Read the model definition and answer for the solid it produces. Units are mm, in the model's axes. Coordinates: 2 decimals unless noted, no trailing zeros. One line per item, written item: value. Start each with the question number.
```python
from build123d import *

# Parameters (mm, degrees)
F0_W     = 127
F0_H     = 127
F0_W_2   = 9.525
F1_DEPTH = 4.7625
F2_D     = 3.556
F3_R     = 3.81


with BuildPart() as f1:
    # F0 (on Top) → F1 (new body)
    with BuildSketch(Plane.XY):
        Rectangle(F0_W, F0_H)
        with Locations((-68.2625, 0)):
            Rectangle(F0_W_2, F0_H)
        with Locations((68.2625, 0)):
            Rectangle(F0_W_2, F0_H)
    extrude(amount=F1_DEPTH)

    # F2 (through all)
    with Locations(Plane(origin=(0, 0, 0), x_dir=(1, 0, 0), z_dir=(0, 0, -1))):
        with Locations((-68.2498, -58.547), (-58.547, -58.547), (-68.2498, -39.497), (-68.2498, 39.497), (-68.2498, 58.547), (-58.547, 58.547), (58.547, 58.547), (68.2625, 58.547), (68.2625, -58.547), (68.2625, -39.497), (58.547, -58.547)):
            Hole(F2_D / 2)

    # F3
    f3_edges = [f1.edges().sort_by_distance(p)[0] for p in [
        (-73.025, 63.5, 2.38125),
        (-73.025, -63.5, 2.38125),
        (73.025, -63.5, 2.38125),
        (73.025, 63.5, 2.38125),
    ]]
    fillet(f3_edges, radius=F3_R)


solid = f1.part
```
1) A flat-ended cylindrical pin translates along its axis: pin 1 (5.5 mm diameter, centred on x = 68.26, y = -58.55, fed in from +Z). Find the tip coordinate at first contact, or state that the pin passes through.
2) Consider line 1 along X through (y, z) = (-57, 0.25) (3 decimals); line 2 along Y through (x, z) = (58, 0.5); line 3 along Y through (x, z) = (-59.5, 2.95). Determine where each line is inside the solid, lowest interval first.
3) For a pull along Y with two mould halves and no side action, classify faces 1 (the face through (-1, 1, 0)), 2 (the face through (-71.94, 62.35, 2.41)), 3 (the face through (-69.946, -59.081, 2.415)) as released by +Y, released by -Y, zero draft, split by the parting line, or undercut.
Results found:
1. pin 1: stops at z = 4.76
2. line 1: x = -73.025 to -69.126, -67.373 to -59.423, -57.671 to 57.671, 59.423 to 67.386, 69.139 to 73.025
2. line 2: y = -63.5 to -60.24, -56.86 to 56.86, 60.24 to 63.5
2. line 3: y = -63.5 to -60.05, -57.05 to 57.05, 60.05 to 63.5
3. face 1: zero draft
3. face 2: released by +Y
3. face 3: undercut
